The listing builds one solid part. Answer for the finished solid, in the listing's coordinates (mm). A direction names the side the tool comes from. Round coordinates to 2 decimals unless told otherwise and drop trailing zeros. Loops run counter-clockwise (first coordinate to the right, second up) from the corner with the lowest first, then second, coordinate; pieces in that order, holes last. Notation, with made-up numbers: (14.5, 49.25) - (52.5, 49.25) arc R21 cw to (52.5, 78.25) - close; hole circle Ø2 at (-21, 4). An arc over 180 degrees is marked (long way). One line per item, written item: value.
```python
from build123d import *

# Parameters (mm, degrees)
SKETCH_W        = 180
SKETCH_H        = 100
PAD_DEPTH       = 55
THICKNESS_T     = -3
SKETCH001_R     = 4
POCKET_DEPTH    = 16
PAD004_START    = -8
SKETCH005_W     = 8
SKETCH005_H     = 8
SKETCH005_R     = 1.5
PAD004_DEPTH    = 49
SKETCH008_W     = 2
SKETCH008_H     = 8
POCKET002_DEPTH = 3
FILLET_R        = 3
FILLET001_R     = 3


with BuildPart() as part:
    # Sketch (on XY_Plane of Origin) → Pad (new body)
    with BuildSketch(Plane.XY):
        with Locations((90, 50)):
            Rectangle(SKETCH_W, SKETCH_H)
    extrude(amount=PAD_DEPTH)

    # Thickness
    thickness_openings = [part.faces().sort_by_distance(p)[0] for p in [
        (90, 50, 55),
    ]]
    offset(amount=THICKNESS_T, openings=thickness_openings)

    # Sketch001 (on YZ_Plane of Origin) → Pocket (cut)
    with BuildSketch(Plane.YZ):
        with Locations((43, 9)):
            Circle(SKETCH001_R)
    extrude(amount=POCKET_DEPTH, mode=Mode.SUBTRACT)

    # Sketch005 → Pad004 (join)
    with BuildSketch(Plane.XY.offset(60).offset(PAD004_START)):
        with Locations((7, 93)):
            Rectangle(SKETCH005_W, SKETCH005_H)
        with Locations((7, 93)):
            Circle(SKETCH005_R, mode=Mode.SUBTRACT)
        with Locations((173, 7)):
            Rectangle(SKETCH005_W, SKETCH005_H)
        with Locations((173, 7)):
            Circle(SKETCH005_R, mode=Mode.SUBTRACT)
        with Locations((173, 93)):
            Rectangle(SKETCH005_W, SKETCH005_H)
        with Locations((173, 93)):
            Circle(SKETCH005_R, mode=Mode.SUBTRACT)
        with Locations((7, 7)):
            Rectangle(SKETCH005_W, SKETCH005_H)
        with Locations((7, 7)):
            Circle(SKETCH005_R, mode=Mode.SUBTRACT)
    extrude(amount=-PAD004_DEPTH)

    # Sketch008 (on Face14 of Pad004) → Pocket002 (cut)
    with BuildSketch(Plane.XY.offset(3)):
        with Locations((148, 78)):
            Rectangle(SKETCH008_W, SKETCH008_H)
    extrude(amount=-POCKET002_DEPTH, mode=Mode.SUBTRACT)

    # Fillet
    fillet_edges = [part.edges().sort_by_distance(p)[0] for p in [
        (11, 11, 27.5),
        (169, 11, 27.5),
        (169, 89, 27.5),
        (11, 89, 27.5),
    ]]
    fillet(fillet_edges, radius=FILLET_R)

    # Fillet001
    fillet001_edges = [part.edges().sort_by_distance(p)[0] for p in [
        (180, 0, 27.5),
        (180, 100, 27.5),
        (0, 0, 27.5),
        (0, 100, 27.5),
    ]]
    fillet(fillet001_edges, radius=FILLET001_R)


solid = part.part
```
1) A cutting plane is placed at C-C on x = 26. Give the vertices of the cut face in (y, z).
Final values:
outline: (0, 0) - (100, 0) - (100, 55) - (97, 55) - (97, 3) - (3, 3) - (3, 55) - (0, 55) - close
2) A cutting plane is placed at D-D on y = 53. Give the vertices of the cut face in (x, z).
Final values:
outline: (0, 0) - (180, 0) - (180, 55) - (177, 55) - (177, 3) - (3, 3) - (3, 55) - (0, 55) - close
3) For faces 4 (the flat face through (175, 7, 52)), 5 (the flat face through (180, 49, 27)), determine the directions among +Z, -Z, +X, -X, +Y, -Y from which every point of the face is accessible in a straight line to the end or side of a thin tool.
Final values:
face 4: +Z
face 5: +Z, -Z, +X, +Y, -Y
4) Consider L1, parallel to X at y = 93, z = 21; L2, parallel to Y at x = 173, z = 28; L3, parallel to Z at x = 2, y = 43. Determine where each line is inside the solid, lowest interval first.
Final values:
L1: 0 to 5.5, 8.5 to 11, 169 to 171.5, 174.5 to 180
L2: 0 to 5.5, 8.5 to 11, 89 to 91.5, 94.5 to 100
L3: 0 to 5, 13 to 55
5) For a pull along Z with two mould halves and no side action, classify faces 1 (the flat face through (63, 2, 55)), 2 (the flat face through (169, 94, 28)), 3 (the cylindrical face through (1.5, 39.8, 6.6)) as released by +Z, released by -Z, zero draft, split by the parting line, or undercut.
Final values:
face 1: released by +Z
face 2: zero draft
face 3: undercut
6) Each of these flat-tipped pins is pushed along its axis until it touches: pin 1 Ø3.5 at (x, y) = (173, 93) entering from +Z; pin 2 Ø6 at (x, y) = (105.5, 51.5) entering from +Z. Where does it stop, or does it pass through?
Final values:
pin 1: z = 52
pin 2: z = 3
7) A cutting plane is placed at A-A on y = 43. Give the vertices of the cut face in (x, z), and give its area (3 significant figures).
Final values:
outline: (0, 0) - (180, 0) - (180, 55) - (177, 55) - (177, 3) - (3, 3) - (3, 5) - (0, 5) - close; (0, 13) - (3, 13) - (3, 55) - (0, 55) - close
area: 828 mm2
8) A cutting plane is placed at B-B on z = 38. Give the vertices of the cut face in (x, y), and give its area (3 significant figures).
Final values:
outline: (0, 3) arc R3 ccw to (3, 0) - (177, 0) arc R3 ccw to (180, 3) - (180, 97) arc R3 ccw to (177, 100) - (3, 100) arc R3 ccw to (0, 97) - close; hole (3, 11) - (8, 11) arc R3 cw to (11, 8) - (11, 3) - (169, 3) - (169, 8) arc R3 cw to (172, 11) - (177, 11) - (177, 89) - (172, 89) arc R3 cw to (169, 92) - (169, 97) - (11, 97) - (11, 92) arc R3 cw to (8, 89) - (3, 89) - close; hole circle Ø3 at (7, 7); hole circle Ø3 at (7, 93); hole circle Ø3 at (173, 7); hole circle Ø3 at (173, 93)
area: 1,860 mm2
